```python
from build123d import *

# Parameters (mm, degrees)
F1_DEPTH = 35


with BuildPart() as f1:
    # F0 (on Front) → F1 (new body)
    with BuildSketch(Plane.XZ):
        with BuildLine():
            Line((12.085786, 0), (0, 0))
            Line((0, 0), (0, -0.5))
            Line((0, -0.5), (12.085786, -0.5))
            Line((12.085786, -0.5), (31.724476, -0.5))
            ThreePointArc((31.724476, -0.5), (32.080347, -0.64878), (32.224432, -1.006578))
            Line((32.224432, -1.006578), (32.197876, -3.025085))
            Line((32.197876, -3.025085), (31.25063, -75.025085))
            ThreePointArc((31.25063, -75.025085), (30.612597, -75.944154), (29.521571, -75.696289))
            Line((29.521571, -75.696289), (26.838608, -72.729523))
            Line((26.838608, -72.729523), (26.467762, -73.064893))
            Line((26.467762, -73.064893), (29.150726, -76.03166))
            ThreePointArc((29.150726, -76.03166), (30.771804, -76.436713), (31.761848, -75.090692))
            Line((31.761848, -75.090692), (32.697247, -3.05017))
            Line((32.697247, -3.05017), (32.723698, -1.012983))
            ThreePointArc((32.723698, -1.012983), (32.435465, -0.297498), (31.723783, 0))
            Line((31.723783, 0), (12.085786, 0))
        make_face()
        with BuildLine():
            Line((0, -0.5), (0, 0))
            Line((0, 0), (-12.085786, 0))
            Line((-12.085786, 0), (-31.723783, 0))
            ThreePointArc((-31.723783, 0), (-32.435465, -0.297498), (-32.723698, -1.012983))
            Line((-32.723698, -1.012983), (-32.697247, -3.05017))
            Line((-32.697247, -3.05017), (-31.761848, -75.090692))
            ThreePointArc((-31.761848, -75.090692), (-30.771804, -76.436713), (-29.150726, -76.03166))
            Line((-29.150726, -76.03166), (-26.467762, -73.064893))
            Line((-26.467762, -73.064893), (-26.838608, -72.729523))
            Line((-26.838608, -72.729523), (-29.521571, -75.696289))
            ThreePointArc((-29.521571, -75.696289), (-30.612597, -75.944154), (-31.25063, -75.025085))
            Line((-31.25063, -75.025085), (-32.197876, -3.025085))
            Line((-32.197876, -3.025085), (-32.224432, -1.006578))
            ThreePointArc((-32.224432, -1.006578), (-32.080347, -0.64878), (-31.724476, -0.5))
            Line((-31.724476, -0.5), (-12.085786, -0.5))
            Line((-12.085786, -0.5), (0, -0.5))
        make_face()
    extrude(amount=F1_DEPTH)


solid = f1.part
```
Could you check a few things on this model? Use its own coordinates, in mm. A direction names the side the tool comes from. Round coordinates to 2 decimals unless told otherwise and drop trailing zeros. Loops run counter-clockwise (first coordinate to the right, second up) from the corner with the lowest first, then second, coordinate; pieces in that order, holes last. Notation, with made-up numbers: (37, 10.5) -> (74, 10.5) arc R30 ccw to (74, 36.5) -> close; hole circle Ø6 at (80, 78.5). An arc over 180 degrees is marked (long way). Put each result on its own line as item: value.
Q1. For pin 1 Ø5 at (x, y) = (21, -27) entering from -Z; pin 2 Ø5 at (y, z) = (-13, -25.5) entering from +X; pin 3 Ø10 at (y, z) = (-23.5, -8) entering from +X, each with a flat end and sliding along its axis, tell me the tip position at first contact or that it passes through.
Checks:
pin 1: z = -0.5
pin 2: x = 32.44
pin 3: x = 32.7
Q2. I want a section at B-B on y = -6. Write out the boundary of the cut face in (x, z).
Checks:
outline: (-32.72, -1.01) -> (-32.7, -3.05) -> (-31.76, -75.09) arc R1.5 ccw to (-29.15, -76.03) -> (-26.47, -73.06) -> (-26.84, -72.73) -> (-29.52, -75.7) arc R1 cw to (-31.25, -75.03) -> (-32.22, -1.01) arc R0.5 cw to (-31.72, -0.5) -> (31.72, -0.5) arc R0.5 cw to (32.22, -1.01) -> (31.25, -75.03) arc R1 cw to (29.52, -75.7) -> (26.84, -72.73) -> (26.47, -73.06) -> (29.15, -76.03) arc R1.5 ccw to (31.76, -75.09) -> (32.7, -3.05) -> (32.72, -1.01) arc R1 ccw to (31.72, 0) -> (-31.72, 0) arc R1 ccw to start
Q3. Please list where these lines run through material, in increasing order: line 1 (Z direction, x = 26, y = -15); line 2 (Z direction, x = -27, y = -23); line 3 (X direction, y = -30, z = -18.5). Write a range as from..to.
Checks:
line 1: -0.5..0
line 2: -73.65..-72.91, -0.5..0
line 3: -32.5..-31.99, 31.99..32.5
Q4. Thinking about a two-plate mould opening in X: for faces 1 (the cylindrical face through (-30.795, -17.255, -76.428)), 2 (the flat face through (-31.7, 0, -60.8)), which applies, pulls with the +X half, pulls with the -X half, needs draft (parallel to the pull), parting line crosses it, or undercut?
Checks:
face 1: undercut
face 2: needs draft
Q5. Which directions (+Z, -Z, +X, -X, +Y, -Y) give clear straight access to the entire face, cutting with the end or side of a thin tool? Please do faces 3 (the flat face through (0, -17, 0)), 4 (the cylindrical face through (-30.6, -17.26, -75.95)), 5 (the flat face through (27.79, -17.255, -74.528)).
Checks:
face 3: +Z, +X, -X, +Y, -Y
face 4: +Y, -Y
face 5: -Z, +Y, -Y
Q6. I want a section at C-C on x = -21.5. Write out the boundary of the cut face in (y, z), and give its area (3 significant figures).
Checks:
outline: (-35, -0.5) -> (0, -0.5) -> (0, 0) -> (-35, 0) -> close
area: 17.5 mm2
Q7. I want a section at A-A on z = -9. Write out the boundary of the cut face in (x, y), and give its area (3 significant figures).
Checks:
outline: (-32.62, -35) -> (-32.12, -35) -> (-32.12, 0) -> (-32.62, 0) -> close; (32.12, -35) -> (32.62, -35) -> (32.62, 0) -> (32.12, 0) -> close
area: 35.1 mm2
